from build123d import *

# Parameters (mm, degrees)
BOSS_EXTRUDE5_DEPTH  = 5
SKETCH3_W            = 50
SKETCH3_H            = 11
BOSS_EXTRUDE6_DEPTH  = 50
SKETCH5_R            = 2.25
CUT_EXTRUDE1_DEPTH   = 11
BOSS_EXTRUDE8_DEPTH  = 10
CUT_EXTRUDE2_DEPTH   = 10
SKETCH8_W            = 2
SKETCH8_H            = 15.993233409
CUT_EXTRUDE3_DEPTH   = 5
SKETCH9_W            = 10
SKETCH9_H            = 10
BOSS_EXTRUDE9_DEPTH  = 10
SKETCH10_W           = 10
SKETCH10_H           = 10
BOSS_EXTRUDE10_DEPTH = 10
FILLET1_R            = 10
FILLET2_R            = 5
SKETCH11_W           = 15.1
SKETCH11_H           = 10
BOSS_EXTRUDE11_DEPTH = 2
SKETCH12_W           = 60.2
SKETCH12_H           = 10
BOSS_EXTRUDE12_DEPTH = 2
BOSS_EXTRUDE14_REACH = 84.491
SKETCH14_W           = 49.873600962
SKETCH14_H           = 10
FILLET3_R            = 1
SKETCH15_W           = 46
SKETCH15_H           = 5
BOSS_EXTRUDE15_DEPTH = 22


with BuildPart() as part:
    # Sketch1 → Boss-Extrude5 (new body)
    with BuildSketch(Plane(origin=(0, 0, 0), x_dir=(1, 0, 0), z_dir=(0, 1, 0))):
        Polygon((-25, 20), (25, 20), (25, 0), (25, -6.94447706), (-25, -6.94447706), (-25, 0.55552294), align=None)
    extrude(amount=BOSS_EXTRUDE5_DEPTH)

    # Sketch3 → Boss-Extrude6 (add)
    with BuildSketch(Plane.XZ):
        with Locations((0, 1.44447706)):
            Rectangle(SKETCH3_W, SKETCH3_H)
    extrude(amount=BOSS_EXTRUDE6_DEPTH)

    # Sketch5 → Cut-Extrude1 (cut)
    with BuildSketch(Plane.XY.offset(6.94447706)):
        with Locations((-20.5, -45)):
            Circle(SKETCH5_R)
        with Locations(Location((-20.5, -37, 0), (0, 0, 180))):
            Circle(SKETCH5_R)
        with Locations(Location((-12.5, -45, 0), (0, 0, 180))):
            Circle(SKETCH5_R)
        with Locations((-12.5, -37)):
            Circle(SKETCH5_R)
        with Locations((12.5, -45)):
            Circle(SKETCH5_R)
        with Locations(Location((20.5, -45, 0), (0, 0, 180))):
            Circle(SKETCH5_R)
        with Locations(Location((12.5, -37, 0), (0, 0, 180))):
            Circle(SKETCH5_R)
        with Locations((20.5, -37)):
            Circle(SKETCH5_R)
    extrude(amount=-CUT_EXTRUDE1_DEPTH, mode=Mode.SUBTRACT)

    # Sketch6 → Boss-Extrude8 (add)
    with BuildSketch(Plane(origin=(0, 0, -4.05552294), x_dir=(-1, 0, 0), z_dir=(0, 0, -1))):
        Polygon((-25, -11.208830651), (25, -11.208830651), (60, -11.208830651), (60, -21.208830651), (25, -21.208830651), (-25, -21.208830651), (-60, -21.208830651), (-60, -11.208830651), align=None)
    extrude(amount=BOSS_EXTRUDE8_DEPTH)

    # Sketch7 → Cut-Extrude2 (cut)
    with BuildSketch(Plane.XY.offset(-4.05552294)):
        Polygon((30.1, -21.208830651), (30.1, -19.929430473), (25.639200757, -19.929430473), (25.639200757, -18.229430473), (30.1, -18.229430473), (30.1, -14.208830651), (54.9, -14.208830651), (54.9, -18.229430473), (59.360799243, -18.229430473), (59.360799243, -19.929430473), (54.9, -19.929430473), (54.9, -21.208830651), align=None)
        Polygon((-25.639200757, -19.929430473), (-25.639200757, -18.229430473), (-30.1, -18.229430473), (-30.1, -14.208830651), (-54.9, -14.208830651), (-54.9, -18.229430473), (-59.360799243, -18.229430473), (-59.360799243, -19.929430473), (-54.9, -19.929430473), (-54.9, -21.208830651), (-30.1, -21.208830651), (-30.1, -19.929430473), align=None)
    extrude(amount=-CUT_EXTRUDE2_DEPTH, mode=Mode.SUBTRACT)

    # Sketch8 → Cut-Extrude3 (cut)
    with BuildSketch(Plane(origin=(0, 5, 0), x_dir=(1, 0, 0), z_dir=(0, 1, 0))):
        with Locations((-24, 12.003383296)):
            Rectangle(SKETCH8_W, SKETCH8_H)
        with Locations((24, 12.003383296)):
            Rectangle(SKETCH8_W, SKETCH8_H)
    extrude(amount=-CUT_EXTRUDE3_DEPTH, mode=Mode.SUBTRACT)

    # Sketch9 → Boss-Extrude9 (add)
    with BuildSketch(Plane.ZY.offset(60)):
        with Locations((-9.05552294, -16.208830651)):
            Rectangle(SKETCH9_W, SKETCH9_H)
    extrude(amount=BOSS_EXTRUDE9_DEPTH)

    # Sketch10 → Boss-Extrude10 (add)
    with BuildSketch(Plane(origin=(60, 0, 0), x_dir=(0, 0, -1), z_dir=(1, 0, 0))):
        with Locations((9.05552294, -16.208830651)):
            Rectangle(SKETCH10_W, SKETCH10_H)
    extrude(amount=BOSS_EXTRUDE10_DEPTH)

    # Fillet1
    fillet1_edges = [part.edges().sort_by_distance(p)[0] for p in [
        (0, 5, 6.94447706),
    ]]
    fillet(fillet1_edges, radius=FILLET1_R)

    # Fillet2
    fillet2_edges = [part.edges().sort_by_distance(p)[0] for p in [
        (-70, -11.208830651, -9.05552294),
        (70, -11.208830651, -9.05552294),
        (-25, -50, 1.44447706),
        (25, -50, 1.44447706),
    ]]
    fillet(fillet2_edges, radius=FILLET2_R)

    # Sketch11 → Boss-Extrude11 (add)
    with BuildSketch(Plane.XZ.offset(21.208830651)):
        with Locations((62.45, -9.05552294)):
            Rectangle(SKETCH11_W, SKETCH11_H)
        with Locations((-62.45, -9.05552294)):
            Rectangle(SKETCH11_W, SKETCH11_H)
    extrude(amount=BOSS_EXTRUDE11_DEPTH)

    # Sketch12 → Boss-Extrude12 (add)
    with BuildSketch(Plane.XZ.offset(21.208830651)):
        with Locations((0, -9.05552294)):
            Rectangle(SKETCH12_W, SKETCH12_H)
    extrude(amount=BOSS_EXTRUDE12_DEPTH)

    # Boss-Extrude14: up to this face of the body (flat: up to its plane)
    boss_extrude14_end = Plane(part.part.faces().sort_by_distance((0, 5, -11.488914502))[0])
    # Sketch14 → Boss-Extrude14 (add, up to the picked face)
    with BuildSketch(Plane(origin=(0, -11.208830651, 0), x_dir=(1, 0, 0), z_dir=(0, 1, 0)), mode=Mode.PRIVATE) as boss_extrude14_sk1:
        with Locations((-0.063199519, 9.05552294)):
            Rectangle(SKETCH14_W, SKETCH14_H)
    boss_extrude14_tool1 = split(extrude(boss_extrude14_sk1.sketch, amount=BOSS_EXTRUDE14_REACH, mode=Mode.PRIVATE), bisect_by=boss_extrude14_end, keep=Keep.BOTH, mode=Mode.PRIVATE)
    add(boss_extrude14_tool1.solids().sort_by(Axis((-0.0632, -11.208831, -9.055523), (0, 1, 0)))[0])

    # Fillet3
    fillet3_edges = [part.edges().sort_by_distance(p)[0] for p in [
        (-23, 2.5, -14.05552294),
        (23, 2.5, -14.05552294),
    ]]
    fillet(fillet3_edges, radius=FILLET3_R)

    # Sketch15 → Boss-Extrude15 (add)
    with BuildSketch(Plane(origin=(0, 0, -20), x_dir=(-1, 0, 0), z_dir=(0, 0, -1))):
        with Locations((0, 2.5)):
            Rectangle(SKETCH15_W, SKETCH15_H)
    extrude(amount=BOSS_EXTRUDE15_DEPTH)


solid = part.part
Can you work these out from the model? Positions are in its coordinate system, mm. A direction names the side the tool comes from. Give positions to 0.01 mm unless a question says otherwise; leave off trailing zeros. Order: outer loops, then holes, each group sorted by start corner. A loop starts at its lowest first (then second) coordinate and runs counter-clockwise, first axis right, second up. Notation, with made-up numbers: M 8.25,-35.75 L 38.25,-35.75 A24 cw 38.25,-1.75 Z; hole C 33.25,49.25 d11. An arc over 180 degrees is marked long. Use one line per item in the form item = value. Start each with the question number.
Item 1: If we section it at B-B (x = -57.5): Write out the boundary of the cut face in (y, z).
Item 2: Will these pins go through, and if not, where does the flat tip stop? pin 1 Ø10 at (x, y) = (14.5, -5.5) entering from -Z; pin 2 Ø5 at (y, z) = (-1, -9.5) entering from +X; pin 3 Ø6 at (x, y) = (10, -44.5) entering from -Z.
Item 3: If I drill on line 1 along Y through (x, z) = (-20.5, -0.75); line 2 along Y through (x, z) = (20, 0); line 3 along Z through (x, y) = (-1.5, -7), over which ranges is the centre line in solid material (lowest first)?
Item 4: For faces 5 (the cylindrical face through (-24, -48, 2)), 6 (the flat face through (54.9, -22, -9)), 7 (the flat face through (28, -18.229, -9)), which set-ups out of +Z, -Z, +X, -X, +Y, -Y let a thin tool reach every point of the face, with its end or its side?
Item 5: If we section it at D-D (x = 3.5): Write out the boundary of the cut face in (y, z), then the cut area to 3 significant figures.
Item 6: If we section it at C-C (x = -12.5): Write out the boundary of the cut face in (y, z).
Item 7: If we section it at A-A (y = -37): Write out the boundary of the cut face in (x, z), then the cut area to 3 significant figures.
Item 8: We'd pull the mould along X, two halves only. Please class faces 1 (the cylindrical face through (19.29, -46.897, 1.521)), 2 (the flat face through (24.874, -3, -9)), 3 (the flat face through (30.1, -16, -9)), 4 (the flat face through (0, -50, 2)): +X half, -X half, draft (parallel to the pull), parting line (faces both ways), or undercut.
Outcome:
q1.outline = M -23.21,-14.06 L -19.93,-14.06 L -19.93,-4.06 L -23.21,-4.06 Z; M -18.23,-14.06 L -11.21,-14.06 L -11.21,-4.06 L -18.23,-4.06 Z
q2.pin_1 = -14.06
q2.pin_2 = 24.87
q2.pin_3 = -4.06
q3.line_1 = -49.97 to -47.25, -42.75 to -39.25, -34.75 to 4.73
q3.line_2 = -50 to -47.19, -42.81 to -39.19, -34.81 to 4.52
q3.line_3 = -14.06 to 6.94
q4.face_5 = +Z, -Z, -X, -Y
q4.face_6 = +Z, -Z, -Y
q4.face_7 = +Z, -Z
q5.outline = M -50,-4.06 L -23.21,-4.06 L -23.21,-14.06 L 0,-14.06 L 0,-42 L 5,-42 L 5,-3.06 A10 ccw -5,6.94 L -50,6.94 Z
q5.area = 1,010 mm2
q6.outline = M -50,-4.06 L -47.25,-4.06 L -47.25,6.94 L -50,6.94 Z; M -42.75,-4.06 L -39.25,-4.06 L -39.25,6.94 L -42.75,6.94 Z; M -34.75,-4.06 L -23.21,-4.06 L -23.21,-14.06 L 0,-14.06 L 0,-42 L 5,-42 L 5,-3.06 A10 ccw -5,6.94 L -34.75,6.94 Z
q7.outline = M -25,-4.06 L -22.75,-4.06 L -22.75,6.94 L -25,6.94 Z; M -18.25,-4.06 L -14.75,-4.06 L -14.75,6.94 L -18.25,6.94 Z; M -10.25,-4.06 L 10.25,-4.06 L 10.25,6.94 L -10.25,6.94 Z; M 14.75,-4.06 L 18.25,-4.06 L 18.25,6.94 L 14.75,6.94 Z; M 22.75,-4.06 L 25,-4.06 L 25,6.94 L 22.75,6.94 Z
q7.area = 352 mm2
q8.face_1 = undercut
q8.face_2 = +X half
q8.face_3 = undercut
q8.face_4 = draft
